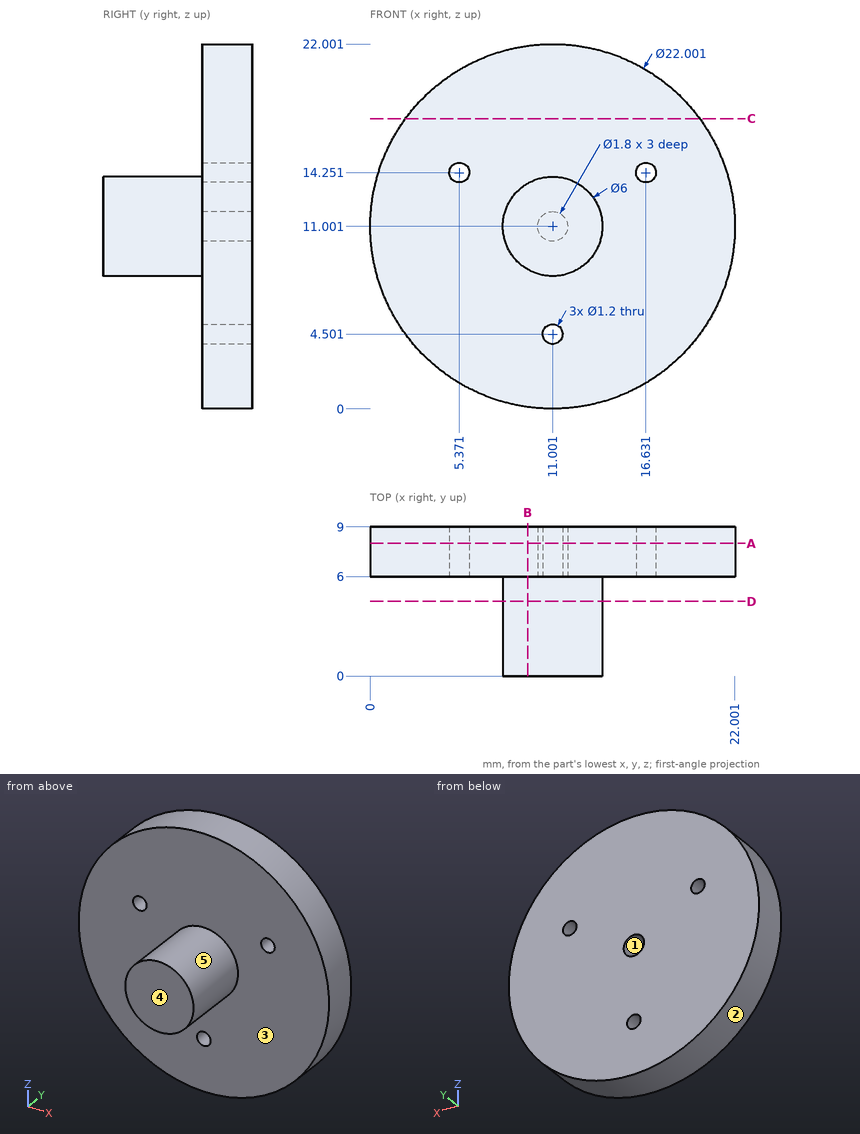
Study the drawing (mm; zero at the part's minimum x, y, z) and answer. A direction names the side the tool comes from. Round coordinates to 2 decimals unless told otherwise and drop trailing zeros. Loops run counter-clockwise (first coordinate to the right, second up) from the corner with the lowest first, then second, coordinate; pieces in that order, holes last. Notation, with made-up numbers: M 42.5,23.25 L 46.5,23.25 A22 ccw 46.5,54.25 Z; hole C 27.25,52.5 d1. An arc over 180 degrees is marked long. One line per question, with ' | ' between items.
Q1. The mould has two halves that part along Z. Classify the marked faces 1, 2 and 3: +Z half, -Z half, draft (parallel to the pull), parting line (faces both ways), or undercut.
Conclusion:
face 1: undercut | face 2: parting line | face 3: draft
Q2. Find section B-B, the plane x = 9.5. Give the vertices of the cut face in (y, z).
Conclusion:
outline: M 0,8.4 L 6,8.4 L 6,0.1 L 9,0.1 L 9,21.9 L 6,21.9 L 6,13.6 L 0,13.6 Z
Q3. Consider line 1 along Y through (x, z) = (16, 11.25); line 2 along X through (y, z) = (4.25, 8.75) (1 decimal); line 3 along Z through (x, y) = (17.75, 8) (1 decimal). Determine where each line is inside the solid, lowest interval first. Write a range as from..to.
Conclusion:
line 1: y = 6..9 | line 2: x = 9..13 | line 3: z = 2.3..19.7
Q4. Find section C-C, the plane z = 17.5. Give the vertices of the cut face in (x, y) (1 decimal).
Conclusion:
outline: M 2.1,6 L 19.9,6 L 19.9,9 L 2.1,9 Z
Q5. Each of these flat-tipped pins is pushed along its axis until it touches: pin 1 Ø1.1 at (x, z) = (11, 4.5) entering from -Y; pin 2 Ø1.4 at (x, z) = (5.37, 14.25) entering from -Y. Where does it stop, or does it pass through?
Conclusion:
pin 1: passes through | pin 2: stops at y = 6
Q6. Find section D-D, the plane y = 4.5. Give the vertices of the cut face in (x, z).
Conclusion:
outline: C 11,11 d6
Q7. Find section A-A, the plane y = 8. Give the vertices of the cut face in (x, z), then the cut area to 3 significant figures.
Conclusion:
outline: C 11,11 d22; hole C 5.37,14.25 d1.2; hole C 11,11 d1.8; hole C 11,4.5 d1.2; hole C 16.63,14.25 d1.2 | area: 374 mm2
Q8. A tool of negligible diameter and unlimited length cuts with its end or side. For the marked faces 4 and 5, from which of +Z, -Z, +X, -X, +Y, -Y can it reach the whole face along a straight path? Write none if from no direction.
Conclusion:
face 4: +Z, -Z, +X, -X, -Y | face 5: -Y
